from build123d import *

# Parameters (mm, degrees)
SKETCH1_W           = 70
SKETCH1_H           = 60
BOSS_EXTRUDE1_DEPTH = 1
SKETCH2_W           = 70
SKETCH2_H           = 60
SKETCH2_W_2         = 66
SKETCH2_H_2         = 56
BOSS_EXTRUDE2_DEPTH = 17.46
SKETCH3_W           = 66
SKETCH3_H           = 56
SKETCH3_W_2         = 56
SKETCH3_H_2         = 46
BOSS_EXTRUDE4_DEPTH = 2
SKETCH4_W           = 13.208
SKETCH4_H           = 11.6586
CUT_EXTRUDE2_DEPTH  = 10
SKETCH8_W           = 56
SKETCH8_H           = 5
BOSS_EXTRUDE5_DEPTH = 2
SKETCH9_W           = 5
SKETCH9_H           = 20.5
CUT_EXTRUDE3_DEPTH  = 2
SKETCH13_W          = 68.2
SKETCH13_H          = 58.2
SKETCH13_W_2        = 66
SKETCH13_H_2        = 56
CUT_EXTRUDE6_DEPTH  = 5
FILLET1_R           = 0.8
FILLET2_R           = 0.8


with BuildPart() as part:
    # Sketch1 → Boss-Extrude1 (new body)
    with BuildSketch(Plane(origin=(0, 0, 0), x_dir=(1, 0, 0), z_dir=(0, 1, 0))):
        with Locations((12.443609023, -14.445488722)):
            Rectangle(SKETCH1_W, SKETCH1_H)
    extrude(amount=BOSS_EXTRUDE1_DEPTH)

    # Sketch2 → Boss-Extrude2 (add)
    with BuildSketch(Plane(origin=(0, 1, 0), x_dir=(1, 0, 0), z_dir=(0, 1, 0))):
        with Locations((12.443609023, -14.445488722)):
            Rectangle(SKETCH2_W, SKETCH2_H)
        with Locations((12.443609023, -14.445488722)):
            Rectangle(SKETCH2_W_2, SKETCH2_H_2, mode=Mode.SUBTRACT)
    extrude(amount=BOSS_EXTRUDE2_DEPTH)

    # Sketch3 → Boss-Extrude4 (add)
    with BuildSketch(Plane(origin=(0, 1, 0), x_dir=(1, 0, 0), z_dir=(0, 1, 0))):
        with Locations((12.443609023, -14.445488722)):
            Rectangle(SKETCH3_W, SKETCH3_H)
        with Locations((12.443609023, -14.445488722)):
            Rectangle(SKETCH3_W_2, SKETCH3_H_2, mode=Mode.SUBTRACT)
    extrude(amount=BOSS_EXTRUDE4_DEPTH)

    # Sketch4 → Cut-Extrude2 (cut)
    with BuildSketch(Plane(origin=(0, 0, -15.554511278), x_dir=(-1, 0, 0), z_dir=(0, 0, -1))):
        Polygon((3.722393626, 18.464576877), (3.722393626, 6.205976877), (3.722393626, 5.005976877), (17.530393626, 5.005976877), (17.530393626, 6.205976877), (17.530393626, 18.464576877), align=None)
        with Locations((10.626393626, 12.335276877)):
            Rectangle(SKETCH4_W, SKETCH4_H, mode=Mode.SUBTRACT)
    extrude(amount=-CUT_EXTRUDE2_DEPTH, mode=Mode.SUBTRACT)


with BuildPart() as cut_extrude2_kept_piece:
    # of the separate pieces the step leaves, the one the design keeps (cut_extrude2_pieces_kept)
    add(part.part.solids().sort_by_distance((-22.556390977, 0, -15.554511278))[0])

    # Sketch8 → Boss-Extrude5 (add)
    with BuildSketch(Plane(origin=(0, 1, 0), x_dir=(1, 0, 0), z_dir=(0, 1, 0))):
        with Locations((12.443609023, -14.445488722)):
            Rectangle(SKETCH8_W, SKETCH8_H)
    extrude(amount=BOSS_EXTRUDE5_DEPTH)

    # Sketch9 → Cut-Extrude3 (cut)
    with BuildSketch(Plane(origin=(0, 3, 0), x_dir=(1, 0, 0), z_dir=(0, 1, 0))):
        with Locations((42.943609023, -27.195488722)):
            Rectangle(SKETCH9_W, SKETCH9_H)
    extrude(amount=-CUT_EXTRUDE3_DEPTH, mode=Mode.SUBTRACT)

    # Sketch13 → Cut-Extrude6 (cut)
    with BuildSketch(Plane(origin=(0, 18.46, 0), x_dir=(1, 0, 0), z_dir=(0, 1, 0))):
        with Locations((12.443609023, -14.445488722)):
            Rectangle(SKETCH13_W, SKETCH13_H)
        with Locations((12.443609023, -14.445488722)):
            Rectangle(SKETCH13_W_2, SKETCH13_H_2, mode=Mode.SUBTRACT)
    extrude(amount=-CUT_EXTRUDE6_DEPTH, mode=Mode.SUBTRACT)

    # Fillet1
    fillet1_edges = [cut_extrude2_kept_piece.edges().sort_by_distance(p)[0] for p in [
        (12.443609023, 0, 44.445488722),
        (47.443609023, 0, 14.445488722),
        (12.443609023, 0, -15.554511278),
        (-22.556390977, 0, 14.445488722),
    ]]
    fillet(fillet1_edges, radius=FILLET1_R)

    # Fillet2
    fillet2_edges = [cut_extrude2_kept_piece.edges().sort_by_distance(p)[0] for p in [
        (-17.530393626, 11.732988439, -15.554511278),
        (-10.626393626, 5.005976877, -15.554511278),
        (-3.722393626, 11.732988439, -15.554511278),
    ]]
    fillet(fillet2_edges, radius=FILLET2_R)


solid = cut_extrude2_kept_piece.part
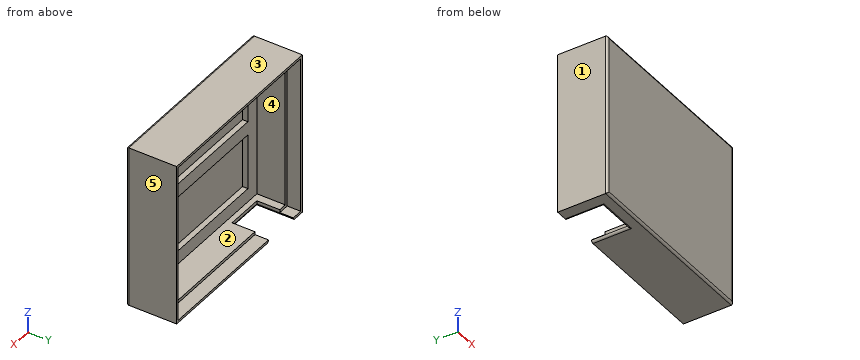
Here's how the part is built. I have some questions about the finished solid (model axes, mm). Face numbers are marked on the shaded views. A direction names the side the tool comes from. Round coordinates to 2 decimals unless told otherwise and drop trailing zeros. Write each loop counter-clockwise with the first axis right and the second up, starting at its lowest first coordinate (ties: lowest second). Pieces come first, ordered by that corner, then holes. Notation, with made-up numbers: (46, 62.25) -> (79, 62.25) arc R14 cw to (79, 70.25) -> close; hole circle Ø8 at (38.25, -18.75). An arc over 180 degrees is marked (long way). One line per item, written item: value.
1) I'm going to push flat-ended pins straight in: pin 1 Ø16.5 at (x, z) = (10.5, 3) entering from +Y; pin 2 Ø1.3 at (x, z) = (-8, -14.5) entering from +Y; pin 3 Ø10 at (x, z) = (-9, 14.5) entering from +Y. Where does each tip first touch, or does it pass through?
Filled sheet:
pin 1: stops at y = 1
pin 2: stops at y = 5.01
pin 3: stops at y = 3
2) Suppose I cut it at D-D on z = 14. List the corners of the cut face in (x, y) for me.
Filled sheet:
outline: (-22.56, 0.8) arc R0.8 ccw to (-21.76, 0) -> (46.64, 0) arc R0.8 ccw to (47.44, 0.8) -> (47.44, 18.46) -> (46.54, 18.46) -> (46.54, 13.46) -> (45.44, 13.46) -> (45.44, 3) -> (-20.56, 3) -> (-20.56, 13.46) -> (-21.66, 13.46) -> (-21.66, 18.46) -> (-22.56, 18.46) -> close
3) Suppose I cut it at C-C on z = 32. List the corners of the cut face in (x, y) for me.
Filled sheet:
outline: (-22.56, 0.8) arc R0.8 ccw to (-21.76, 0) -> (46.64, 0) arc R0.8 ccw to (47.44, 0.8) -> (47.44, 18.46) -> (46.54, 18.46) -> (46.54, 13.46) -> (45.44, 13.46) -> (45.44, 1) -> (-15.56, 1) -> (-15.56, 3) -> (-20.56, 3) -> (-20.56, 13.46) -> (-21.66, 13.46) -> (-21.66, 18.46) -> (-22.56, 18.46) -> close
4) Suppose I cut it at B-B on y = 8.25. List the corners of the cut face in (x, z) for me.
Filled sheet:
outline: (-22.56, -15.55) -> (-18.33, -15.55) arc R0.8 ccw to (-17.53, -14.75) -> (-17.53, -13.55) -> (-20.56, -13.55) -> (-20.56, 42.45) -> (45.44, 42.45) -> (45.44, -13.55) -> (-3.72, -13.55) -> (-3.72, -14.75) arc R0.8 ccw to (-2.92, -15.55) -> (47.44, -15.55) -> (47.44, 44.45) -> (-22.56, 44.45) -> close
5) Suppose I cut it at A-A on x = -14. List the corners of the cut face in (y, z) for me.
Filled sheet:
outline: (0, -14.75) arc R0.8 ccw to (0.8, -15.55) -> (4.21, -15.55) arc R0.8 ccw to (5.01, -14.75) -> (5.01, -13.55) -> (3, -13.55) -> (3, -8.55) -> (1, -8.55) -> (1, 11.95) -> (3, 11.95) -> (3, 16.95) -> (1, 16.95) -> (1, 37.45) -> (3, 37.45) -> (3, 42.45) -> (13.46, 42.45) -> (13.46, 43.55) -> (18.46, 43.55) -> (18.46, 44.45) -> (0.8, 44.45) arc R0.8 ccw to (0, 43.65) -> close
6) If I drill on line 1 (Z direction, x = -10, y = 3.75); line 2 (Z direction, x = 8, y = 2.75); line 3 (Z direction, x = 16, y = 17.25), over which ranges is the centre line in solid material (lowest first)? Write a range as [from, to].
Filled sheet:
line 1: z = [-15.55, -13.55], [42.45, 44.45]
line 2: z = [-15.55, -8.55], [11.95, 16.95], [37.45, 44.45]
line 3: z = [-15.55, -14.65], [43.55, 44.45]
7) For the marked faces 1 and 2, which set-ups out of +Z, -Z, +X, -X, +Y, -Y let a thin tool reach every point of the face, with its end or its side?
Filled sheet:
face 1: +Z, -Z, -X, +Y, -Y
face 2: +Y
8) We'd pull the mould along X, two halves only. Please class the marked faces 3, 4 and 5: released by +X, released by -X, zero draft, split by the parting line, or undercut.
Filled sheet:
face 3: zero draft
face 4: undercut
face 5: released by +X
